from build123d import *

# Parameters (mm, degrees)
SKETCH1_W                 = 30.95625
SKETCH1_H                 = 11.90625
BOSS_EXTRUDE1_DEPTH       = 6.2865
SKETCH2_R                 = 2.38125
CUT_EXTRUDE1_DEPTH        = 4.7625
F_4_40_TAPPED_HOLE1_D     = 2.2606
F_4_40_TAPPED_HOLE1_DEPTH = 8.89
F_4_40_TAPPED_HOLE1_TIP   = 0.679152758


with BuildPart() as part:
    # Sketch1 → Boss-Extrude1 (new body)
    with BuildSketch(Plane(origin=(0, 0, 0), x_dir=(1, 0, 0), z_dir=(0, 1, 0))):
        Rectangle(SKETCH1_W, SKETCH1_H)
    extrude(amount=BOSS_EXTRUDE1_DEPTH)

    # Sketch2 → Cut-Extrude1 (cut)
    with BuildSketch(Plane.XZ):
        Circle(SKETCH2_R)
    extrude(amount=-CUT_EXTRUDE1_DEPTH, mode=Mode.SUBTRACT)

    # #4-40 Tapped Hole1
    with Locations(Plane(origin=(0, 6.2865, 0), x_dir=(-1, 0, 0), z_dir=(0, 1, 0))):
        with Locations((9.402022244, 0), (-9.402022244, 0)):
            Hole(F_4_40_TAPPED_HOLE1_D / 2, depth=F_4_40_TAPPED_HOLE1_DEPTH)
            with Locations((0, 0, -(F_4_40_TAPPED_HOLE1_DEPTH + F_4_40_TAPPED_HOLE1_TIP / 2))):  # 118° drill point
                Cone(0, F_4_40_TAPPED_HOLE1_D / 2, F_4_40_TAPPED_HOLE1_TIP, mode=Mode.SUBTRACT)


solid = part.part
Input: part model. Units: mm. Frame: model coordinates. A direction names the side the tool comes from. Coordinates: 2 decimals unless noted, no trailing zeros. Loops run counter-clockwise (first coordinate to the right, second up) from the corner with the lowest first, then second, coordinate; pieces in that order, holes last. Notation, with made-up numbers: (-35, -33) -> (-9, -33) arc R15 ccw to (-9, -27) -> close; hole circle Ø10 at (-10, 65.25). An arc over 180 degrees is marked (long way). Write item = value, one per line. Start each with the question number.
Item 1: Material intervals for line 1 (Z direction, x = 0, y = 2.15); line 2 (X direction, y = 5.5, z = 1); line 3 (Y direction, x = 1.5, z = 0.25), sorted ascending.
Item 2: Cut plane A-A, the plane z = 0. Return loops of the section in (x, y), plus the area to 3 significant figures.
Item 3: Mould query, pull axis X, two halves, no side actions, for faces 1 (the face through (0, 0, -3)), 2 (the face through (-1.89, 2.35, -1.45)), 3 (the face through (15.478, 3, 0)). Classes: pulls with the +X half, pulls with the -X half, needs draft (parallel to the pull), parting line crosses it, or undercut.
Item 4: Cut plane C-C, the plane x = 0. Return loops of the section in (y, z), plus the area to 3 significant figures.
Item 5: Reachability of faces 4 (the face through (-8.358, 3.099, -0.433)), 5 (the face through (0, 4.762, 0)) from +Z, -Z, +X, -X, +Y, -Y: full face, straight path, thin tool, end or side. Return the list, or none.
Item 6: Cut plane B-B, the plane y = 3.5. Return loops of the section in (x, z), plus the area to 3 significant figures.
Item 7: Cut plane D-D, the plane x = -10. Return loops of the section in (y, z).
Ans:
q1.line_1 = -5.95 to -2.38, 2.38 to 5.95
q1.line_2 = -15.48 to -9.93, -8.88 to 8.88, 9.93 to 15.48
q1.line_3 = 4.76 to 6.29
q2.outline = (-15.48, 0) -> (-10.53, 0) -> (-10.53, 6.29) -> (-15.48, 6.29) -> close; (-8.27, 0) -> (-2.38, 0) -> (-2.38, 4.76) -> (2.38, 4.76) -> (2.38, 0) -> (8.27, 0) -> (8.27, 6.29) -> (-8.27, 6.29) -> close; (10.53, 0) -> (15.48, 0) -> (15.48, 6.29) -> (10.53, 6.29) -> close
q2.area = 144 mm²
q3.face_1 = needs draft
q3.face_2 = undercut
q3.face_3 = pulls with the +X half
q4.outline = (0, -5.95) -> (6.29, -5.95) -> (6.29, 5.95) -> (0, 5.95) -> (0, 2.38) -> (4.76, 2.38) -> (4.76, -2.38) -> (0, -2.38) -> close
q4.area = 52.2 mm²
q5.face_4 = +Y, -Y
q5.face_5 = -Y
q6.outline = (-15.48, -5.95) -> (15.48, -5.95) -> (15.48, 5.95) -> (-15.48, 5.95) -> close; hole circle Ø2.26 at (-9.4, 0); hole circle Ø4.76 at (0, 0); hole circle Ø2.26 at (9.4, 0)
q6.area = 343 mm²
q7.outline = (0, -5.95) -> (6.29, -5.95) -> (6.29, -0.96) -> (0, -0.96) -> close; (0, 0.96) -> (6.29, 0.96) -> (6.29, 5.95) -> (0, 5.95) -> close
